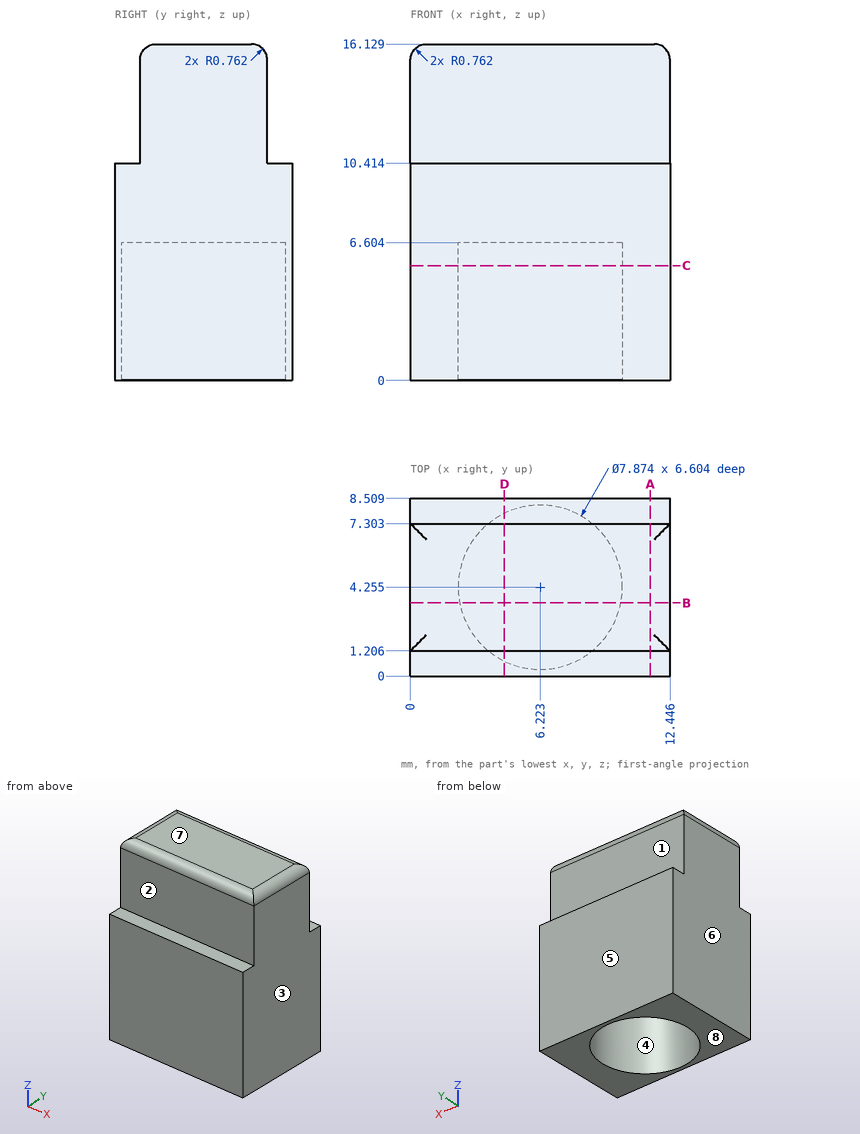
Input: dimensioned drawing with shaded views. Units: mm. Origin: part minimum x, y, z. A direction names the side the tool comes from. Coordinates: 2 decimals unless noted, no trailing zeros. Loops run counter-clockwise (first coordinate to the right, second up) from the corner with the lowest first, then second, coordinate; pieces in that order, holes last. Notation, with made-up numbers: (37.5, 28.5) - (85.5, 28.5) arc R13 cw to (85.5, 35.5) - close; hole circle Ø4 at (59, 81). An arc over 180 degrees is marked (long way). One line per question, with ' | ' between items. Start each with the question number.
(1) Draft query along Z for the marked faces 6, 7 and 8. Return one class per face: +Z half, -Z half, draft (parallel to the pull), parting line (faces both ways), or undercut.
(2) Cut plane C-C on z = 5.5. Output: boundary loops of the cut face in (x, y) (1 decimal).
(3) Cut plane A-A on x = 11.5. Output: boundary loops of the cut face in (y, z) (1 decimal), and give its area (3 significant figures).
(4) First-contact query: pin 1 (2.5 mm diameter, centred on x = 5.5, z = 13.5, fed in from +Y); pin 2 (1 mm diameter, centred on x = 8, y = 8, fed in from +Z); pin 3 (4 mm diameter, centred on x = 7.5, y = 4, fed in from -Z); pin 4 (6 mm diameter, centred on x = 1.5, z = 11.5, fed in from +Y). Flat tips, straight axial feed; report the tip coordinate or a pass-through.
(5) Cut plane D-D on x = 4.5. Output: boundary loops of the cut face in (y, z) (1 decimal).
(6) Reachability of the marked faces 1, 2, 3, 4 and 5 from +Z, -Z, +X, -X, +Y, -Y: full face, straight path, thin tool, end or side. Return the list, or none.
(7) Cut plane B-B on y = 3.5. Output: boundary loops of the cut face in (x, z) (1 decimal).
(8) Ray query, L1, parallel to Z at x = 3, y = 1 (1 decimal); L2, parallel to X at y = 5, z = 5 (1 decimal); L3, parallel to Z at x = 8.25, y = 2.25 (1 decimal). Return the intervals inside material, ascending. Write a range as from..to.
Here are the results:
1) face 6: draft | face 7: +Z half | face 8: -Z half
2) outline: (0, 0) - (12.4, 0) - (12.4, 8.5) - (0, 8.5) - close; hole circle Ø7.9 at (6.2, 4.3)
3) outline: (0, 0) - (8.5, 0) - (8.5, 10.4) - (7.3, 10.4) - (7.3, 15.4) arc R0.8 ccw to (6.5, 16.1) - (2, 16.1) arc R0.8 ccw to (1.2, 15.4) - (1.2, 10.4) - (0, 10.4) - close | area: 123 mm²
4) pin 1: y = 7.3 | pin 2: z = 10.41 | pin 3: z = 6.6 | pin 4: y = 8.51
5) outline: (0, 0) - (0.7, 0) - (0.7, 6.6) - (7.8, 6.6) - (7.8, 0) - (8.5, 0) - (8.5, 10.4) - (7.3, 10.4) - (7.3, 15.4) arc R0.8 ccw to (6.5, 16.1) - (2, 16.1) arc R0.8 ccw to (1.2, 15.4) - (1.2, 10.4) - (0, 10.4) - close
6) face 1: +Z, +X, -X, +Y | face 2: +Z, +X, -X, -Y | face 3: +Z, -Z, +X, +Y, -Y | face 4: -Z | face 5: +Z, -Z, +X, -X, +Y
7) outline: (0, 0) - (2.4, 0) - (2.4, 6.6) - (10.1, 6.6) - (10.1, 0) - (12.4, 0) - (12.4, 15.4) arc R0.8 ccw to (11.7, 16.1) - (0.8, 16.1) arc R0.8 ccw to (0, 15.4) - close
8) L1: 0..10.4 | L2: 0..2.4, 10.1..12.4 | L3: 6.6..16.1
